CAD build for the part. Positions are in the model's coordinates, mm. A direction names the side the tool comes from. Coordinates: 2 decimals unless noted, no trailing zeros. Order: outer loops, then holes, each group sorted by start corner. A loop starts at its lowest first (then second) coordinate and runs counter-clockwise, first axis right, second up. Notation, with made-up numbers: (-24.75, -25.5) - (18.25, -25.5) arc R13 ccw to (18.25, -9.5) - close; hole circle Ø3 at (-15, 78.5). An arc over 180 degrees is marked (long way). Use one line per item in the form item = value.
```python
from build123d import *

# Parameters (mm, degrees)
SZKIC1_R                                 = 4
DODANIE_WYCI_GNI_CIE1_DEPTH              = 20
SZKIC2_OUTSIDE_W                         = 153.84
SZKIC2_OUTSIDE_H                         = 89.84
WYTNIJ_WYCI_GNI_CIE1_DEPTH               = 15
WYTNIJ_WYCI_GNI_CIE2_DEPTH               = 130.135587659
WYTNIJ_WYCI_GNI_CIE2_DEPTH_BACK          = 130.135587659
OTW_R_GWINTOWANY_M8X1_01_D               = 7
OTW_R_GWINTOWANY_M8X1_01_DEPTH           = 9.896987833
OTW_R_GWINTOWANY_M8X1_01_TIP             = 2.103012167
OTW_R_GWINTOWANY_M8X1_01_ON_FACE_2_D     = 7
OTW_R_GWINTOWANY_M8X1_01_ON_FACE_2_DEPTH = 9.896987833
OTW_R_GWINTOWANY_M8X1_01_ON_FACE_2_TIP   = 2.103012167


with BuildPart() as part:
    # Szkic1 → Dodanie-wyciągnięcie1 (new body)
    with BuildSketch(Plane(origin=(0, 0, 0), x_dir=(0, 0, -1), z_dir=(1, 0, 0))):
        with BuildLine():
            Line((-43.138357147, -30), (43.138357147, -30))
            ThreePointArc((43.138357147, -30), (46.738768646, -29.329364235), (49.856267202, -27.407407407))
            ThreePointArc((49.856267202, -27.407407407), (58.828108774, -14.988630917), (62, 0))
            Line((62, 0), (62, 30))
            Line((62, 30), (-62, 30))
            Line((-62, 30), (-62, 0))
            ThreePointArc((-62, 0), (-58.828108774, -14.988630917), (-49.856267202, -27.407407407))
            ThreePointArc((-49.856267202, -27.407407407), (-46.738768646, -29.329364235), (-43.138357147, -30))
        make_face()
        with Locations((-50, 23)):
            Circle(SZKIC1_R, mode=Mode.SUBTRACT)
        with Locations((50, 23)):
            Circle(SZKIC1_R, mode=Mode.SUBTRACT)
        with Locations((50, -17)):
            Circle(SZKIC1_R, mode=Mode.SUBTRACT)
        with Locations((-50, -17)):
            Circle(SZKIC1_R, mode=Mode.SUBTRACT)
        with BuildLine():
            Line((-25, -16), (25, -16))
            ThreePointArc((25, -16), (41, 0), (25, 16))
            Line((25, 16), (-25, 16))
            ThreePointArc((-25, 16), (-41, 0), (-25, -16))
        make_face(mode=Mode.SUBTRACT)
    extrude(amount=DODANIE_WYCI_GNI_CIE1_DEPTH)

    # Szkic2 outside → Wytnij-wyciągnięcie1 (cut)
    # profile 1 of 2: a face of its own
    with BuildSketch(Plane(origin=(20, 0, 0), x_dir=(0, 0, -1), z_dir=(1, 0, 0))):
        Rectangle(SZKIC2_OUTSIDE_W, SZKIC2_OUTSIDE_H)
        with BuildLine():
            Line((21.671768561, 30), (-21.671768561, 30))
            ThreePointArc((-21.671768561, 30), (-26.059642547, 29.512728202), (-30.233707808, 28.074656189))
            ThreePointArc((-30.233707808, 28.074656189), (-48, 0), (-30.233707808, -28.074656189))
            ThreePointArc((-30.233707808, -28.074656189), (-26.059642547, -29.512728202), (-21.671768561, -30))
            Line((-21.671768561, -30), (21.671768561, -30))
            ThreePointArc((21.671768561, -30), (26.059642547, -29.512728202), (30.233707808, -28.074656189))
            ThreePointArc((30.233707808, -28.074656189), (48, 0), (30.233707808, 28.074656189))
            ThreePointArc((30.233707808, 28.074656189), (26.059642547, 29.512728202), (21.671768561, 30))
        make_face(mode=Mode.SUBTRACT)
    # profile 2 of 2: a face of its own
    with BuildSketch(Plane(origin=(20, 0, 0), x_dir=(0, 0, -1), z_dir=(1, 0, 0))):
        with BuildLine():
            Line((-25, -16), (25, -16))
            ThreePointArc((25, -16), (41, 0), (25, 16))
            Line((25, 16), (-25, 16))
            ThreePointArc((-25, 16), (-41, 0), (-25, -16))
        make_face()
    extrude(amount=-WYTNIJ_WYCI_GNI_CIE1_DEPTH, mode=Mode.SUBTRACT)

    # Szkic3 → Wytnij-wyciągnięcie2 (cut, two sides: drawn at the far end of the back side and taken through both)
    with BuildSketch(Plane(origin=(0, 0, -62), x_dir=(-1, 0, 0), z_dir=(0, 0, -1)).offset(-WYTNIJ_WYCI_GNI_CIE2_DEPTH_BACK)):
        Polygon((-20, -30), (-20, 30), (-14.750680188, 30), align=None)
    extrude(amount=WYTNIJ_WYCI_GNI_CIE2_DEPTH + WYTNIJ_WYCI_GNI_CIE2_DEPTH_BACK, mode=Mode.SUBTRACT)

    # Otwór gwintowany M8x1.01
    with Locations(Plane(origin=(15.32718014, 23.410575405, 20), x_dir=(-0.087155742748, 0.996194698092, 0), z_dir=(0.996194698092, 0.087155742748, 0))):
        with Locations((0, 0), (-47, -40), (-47, 0)):
            Hole(OTW_R_GWINTOWANY_M8X1_01_D / 2, depth=OTW_R_GWINTOWANY_M8X1_01_DEPTH)
            with Locations((0, 0, -(OTW_R_GWINTOWANY_M8X1_01_DEPTH + OTW_R_GWINTOWANY_M8X1_01_TIP / 2))):  # 118° drill point
                Cone(0, OTW_R_GWINTOWANY_M8X1_01_D / 2, OTW_R_GWINTOWANY_M8X1_01_TIP, mode=Mode.SUBTRACT)

    # Otwór gwintowany M8x1.01 on face 2
    with Locations(Plane(origin=(15.32718014, 23.410575405, -20), x_dir=(-0.087155971833, 0.996194678049, 0), z_dir=(0.996194678049, 0.087155971833, 0))):
        with Locations((0, 0)):
            Hole(OTW_R_GWINTOWANY_M8X1_01_ON_FACE_2_D / 2, depth=OTW_R_GWINTOWANY_M8X1_01_ON_FACE_2_DEPTH)
            with Locations((0, 0, -(OTW_R_GWINTOWANY_M8X1_01_ON_FACE_2_DEPTH + OTW_R_GWINTOWANY_M8X1_01_ON_FACE_2_TIP / 2))):  # 118° drill point
                Cone(0, OTW_R_GWINTOWANY_M8X1_01_ON_FACE_2_D / 2, OTW_R_GWINTOWANY_M8X1_01_ON_FACE_2_TIP, mode=Mode.SUBTRACT)


solid = part.part
```
Item 1: Two-plate mould, pull along Z, no slides. Class faces 1 (the face through (2.46, -15.19, -58.74)), 2 (the face through (12.6, -29.5, 26.12)), 3 (the face through (10.29, 23.43, -16.53)): +Z half, -Z half, draft (parallel to the pull), parting line (faces both ways), or undercut.
Derived:
face_1 = -Z half
face_2 = +Z half
face_3 = undercut
Item 2: Drill centre lines: line 1 (Z direction, x = 2.7, y = 23); line 2 (Y direction, x = 1.8, z = 50); line 3 (Y direction, x = 7.75, z = -3.5). Where is each one in solid material? Low to high. Write a range as [from, to].
Derived:
line_1 = [-62, -54], [-46, 46], [54, 62]
line_2 = [-27.28, -21], [-13, 19], [27, 30]
line_3 = [-30, -16], [16, 30]
Item 3: Cut at B-B, the plane y = 1.5. Write the cut outline in (x, z).
Derived:
outline = (0, -62) - (5, -62) - (5, -47.96) - (17.24, -47.96) - (17.24, -40.93) - (0, -40.93) - close; (0, 40.93) - (17.24, 40.93) - (17.24, 47.96) - (5, 47.96) - (5, 62) - (0, 62) - close
Item 4: Cut at C-C, the plane z = -39.5. Write the cut outline in (x, y), plus the area to 3 significant figures.
Derived:
outline = (0, -30) - (5, -30) - (5, -21.35) - (19.24, -21.35) - (17.97, -6.76) - (0, -6.76) - close; (0, 6.76) - (16.78, 6.76) - (15.51, 21.35) - (5, 21.35) - (5, 30) - (0, 30) - close
area = 593 mm²
Item 5: Cut at A-A, the plane z = -7. Write the cut outline in (x, y), plus the area to 3 significant figures.
Derived:
outline = (0, -30) - (20, -30) - (18.78, -16) - (0, -16) - close; (0, 16) - (15.98, 16) - (14.75, 30) - (0, 30) - close
area = 487 mm²
Item 6: Drop flat-ended pins along their axis: pin 1 (3 mm diameter, centred on y = -12, z = 43, fed in from +X); pin 2 (3 mm diameter, centred on y = 21.5, z = -44.5, fed in from +X); pin 3 (12 mm diameter, centred on y = -12.5, z = -8, fed in from +X). Give the stop position or say it passes through.
Derived:
pin_1 = 18.56
pin_2 = 5
pin_3 = 18.99
Item 7: 3-axis set-ups, long thin cutter, end or side, ignore diameter. For faces 4 (the face through (9, 0, 41)), 5 (the face through (12.605, -29.526, -25.999)), 6 (the face through (5, 0, -51)): which of +Z, -Z, +X, -X, +Y, -Y reach the whole face in a straight line?
Derived:
face_4 = +X, -X
face_5 = -Z, +X, -Y
face_6 = -Z, +X
Item 8: Cut at D-D, the plane x = 12.5. State how many separate pieces and enclosed holes the cut face has, plus the area to 3 significant figures.
Derived:
separate_pieces = 1
enclosed_holes = 5
area = 2,480 mm²
